Design review of the part built by this model. Coordinates are the model's own, in mm. A direction names the side the tool comes from. Round coordinates to 2 decimals unless told otherwise and drop trailing zeros. Loops run counter-clockwise (first coordinate to the right, second up) from the corner with the lowest first, then second, coordinate; pieces in that order, holes last. Notation, with made-up numbers: (-12, 32) -> (12, 32) arc R9 cw to (12, 45) -> close; hole circle Ø7 at (86, 14.5). An arc over 180 degrees is marked (long way). Answer as CSV lines item,"result". Start each with the question number.
```python
from build123d import *

# Parameters (mm, degrees)
F0_R     = 15.748
F0_R_2   = 12.7
F1_DEPTH = 3.175
F2_DEPTH = 25.4
F3_D     = 19.05


with BuildPart() as f1:
    # F0 (on Front) → F1 (new body)
    with BuildSketch(Plane.XZ):
        Circle(F0_R)
        Circle(F0_R_2, mode=Mode.SUBTRACT)
        Circle(F0_R_2)
    extrude(amount=-F1_DEPTH)

    # F0 (on Front) → F2 (join)
    with BuildSketch(Plane.XZ):
        Circle(F0_R_2)
    extrude(amount=-F2_DEPTH)

    # F3 (through all)
    with Locations(Plane.XZ):
        with Locations((0, 0)):
            Hole(F3_D / 2)


solid = f1.part
```
Q1. To check wall thickness, follow probe 1 along Z at (x, y) = (0, 13.5) (3 decimals); probe 2 along Y at (x, z) = (-6, 14) (3 decimals); probe 3 along X at (y, z) = (4.5, -6.5). State the ranges of each line that lie inside material, in increasing order. Write a range as from..to.
Q2. Add section A-A, the plane z = 0. Give the boundary of the cut face in (x, y) (3 decimals).
Q3. Mouldability with a two-part tool opening along Z and no side actions: class faces 1 (the cylindrical face through (-2.75, 14.13, -12.4)), 2 (the cylindrical face through (7.559, 12.878, -5.796)), 3 (the flat face through (5, 25.4, 9)) as pulls with the +Z half, pulls with the -Z half, needs draft (parallel to the pull), parting line crosses it, or undercut.
Q4. Add section B-B, the plane x = 0. Give the boundary of the cut face in (y, z) (3 decimals), and give its area (3 significant figures).
Q5. Add section D-D, the plane z = 12. Give the boundary of the cut face in (x, y) (3 decimals).
Q6. Machinability: for faces 4 (the flat face through (7, 0, -7)), 5 (the flat face through (-11, 3.175, 7)), which of the approach directions +Z, -Z, +X, -X, +Y, -Y give a long, thin tool a straight path to every point of the face, cutting with its end or side? Answer none if there is none.
Q7. Add section C-C, the plane y = 20.25. Give the boundary of the cut face in (x, z) (3 decimals).
Q8. For pin 1 Ø2 at (x, y) = (11, 17.5) entering from -Z; pin 2 Ø4 at (x, y) = (-3.5, 5.5) entering from +Z; pin 3 Ø5 at (y, z) = (3.5, 6) entering from +X; pin 4 Ø9.5 at (x, z) = (-1, -1.5) entering from +Y, all flat-tipped, find the tip position at first contact; note any pin that passes through.
Worked answers:
1,probe 1,"z = -12.7..-9.525, 9.525..12.7"
1,probe 2,"y = 0..3.175"
1,probe 3,"x = -10.91..-6.96, 6.96..10.91"
2,outline,"(-15.748, 0) -> (-9.525, 0) -> (-9.525, 25.4) -> (-12.7, 25.4) -> (-12.7, 3.175) -> (-15.748, 3.175) -> close; (9.525, 0) -> (15.748, 0) -> (15.748, 3.175) -> (12.7, 3.175) -> (12.7, 25.4) -> (9.525, 25.4) -> close"
3,face 1,"parting line crosses it"
3,face 2,"undercut"
3,face 3,"needs draft"
4,outline,"(0, -15.748) -> (3.175, -15.748) -> (3.175, -12.7) -> (25.4, -12.7) -> (25.4, -9.525) -> (0, -9.525) -> close; (0, 9.525) -> (25.4, 9.525) -> (25.4, 12.7) -> (3.175, 12.7) -> (3.175, 15.748) -> (0, 15.748) -> close"
4,area,"181 mm^2"
5,outline,"(-10.198, 0) -> (10.198, 0) -> (10.198, 3.175) -> (4.158, 3.175) -> (4.158, 25.4) -> (-4.158, 25.4) -> (-4.158, 3.175) -> (-10.198, 3.175) -> close"
6,face 4,"+Z, -Z, +X, -X, -Y"
6,face 5,"+Y"
7,outline,"circle Ø25.4 at (0, 0); hole circle Ø19.05 at (0, 0)"
8,pin 1,"stops at z = -7.83"
8,pin 2,"stops at z = 12.61"
8,pin 3,"stops at x = 15.35"
8,pin 4,"passes through"
